Solid Edge part; units mm, degrees
sketch "Sketch1" plane through (0, 0, 0) normal (0, -1, 0) x (1, 0, 0)
  arc A0 (7.8125, -39.2296) -> (7.8125, 39.2296) centre (0, 0) cw
  arc A1 (7.8125, 39.2296) -> (242.1875, 39.2296) centre (125, 627.6743) ccw
  arc A2 (242.1875, 39.2296) -> (242.1875, -39.2296) centre (250, 0) cw
  arc A3 (242.1875, -39.2296) -> (7.8125, -39.2296) centre (125, -627.6743) ccw
  dimension "D1" = 39.2296
extrude "Protrusion1" add sketch "Sketch1" against normal blind 15
sketch "Sketch2" plane through (125, 0, 0) normal (0, -1, 0) x (1, 0, 0)
  circle A0 centre (125, 0) radius 22
extrude "Cutout1" cut sketch "Sketch2" against normal through all
hole "Agujero_1" at (250, 0, 32.5) direction (0, 1, 0) diameter 6.647 end up to next
pattern_circular "Pattern1" count 6 over 360 about axis through (250, 0, 0) along (0, 1, 0) of "Agujero_1"
sketch "Sketch3" plane through (125, 0, 0) normal (0, -1, 0) x (1, 0, 0)
  circle A0 centre (-125, 0) radius 3.2
extrude "Cutout2" cut sketch "Sketch3" against normal through all
sketch "Sketch4" plane through (125, 15, 0) normal (0, 1, 0) x (1, 0, 0)
  line L0 (-119, -6) -> (-131, -6)
  line L1 (-131, -6) -> (-131, 6)
  line L2 (-131, 6) -> (-119, 6)
  line L3 (-119, 6) -> (-119, -6)
  dimension "D1" = 131
  dimension "D2" = 119
extrude "VaciadoExtruido_3" cut sketch "Sketch4" against normal blind 12
sketch "Sketch5" plane through (125, 15, 0) normal (0, 1, 0) x (1, 0, 0)
  circle A0 centre (-125, 0) radius 20
extrude "VaciadoExtruido_4" cut sketch "Sketch5" against normal blind 3
hole "Agujero_7" at (-13, 0, 0) direction (0, 1, 0) diameter 4.5 end up to next counterbore diameter 8 counterbore depth 7
pattern_circular "Pattern2" count 6 over 360 about axis through (0, 0, 0) along (0, 1, 0) of "Agujero_7"
hole "Agujero_13" at (48.91, 0, 15) direction (0, 1, 0) diameter 6.647 end up to next
hole "Hole11" at (145.41, 0, 15) direction (0, 1, 0) diameter 6.647 end up to next
hole "Hole12" at (145.41, 0, -15) direction (0, 1, 0) diameter 6.647 end up to next
hole "Hole13" at (48.91, 0, -15) direction (0, 1, 0) diameter 6.647 end up to next
sketch "Sketch6" plane through (125, 0, 0) normal (0, -1, 0) x (1, 0, 0)
  line L0 (7.41, -22) -> (-63.09, -22)
  line L1 (-63.09, -22) -> (-63.09, 22)
  line L2 (-63.09, 22) -> (7.41, 22)
  line L3 (7.41, 22) -> (7.41, -22)
  dimension "D1" = 63.09
  dimension "D2" = 7.41
extrude "Cutout3" cut sketch "Sketch6" against normal through all
fillet "Redondeo_1" radius 5 4 edges at (61.91, 7.5, 22) (132.41, 7.5, 22) (61.91, 7.5, -22) (132.41, 7.5, -22)
For this review, take the finished solid that the model builds, in its own axes (mm). A direction names the side the tool comes from. Give positions to 0.01 mm unless a question says otherwise; leave off trailing zeros. Loops run counter-clockwise (first coordinate to the right, second up) from the corner with the lowest first, then second, coordinate; pieces in that order, holes last. Notation, with made-up numbers: M -4,83.25 L 17,83.25 A25 cw 17,105.25 Z; hole C -16.5,-9 d7. An arc over 180 degrees is marked long. Put each result on its own line as item: value. Start each with the question number.
(1) For pin 1 (2 mm diameter, centred on y = 11.5, z = 4, fed in from +X); pin 2 (6 mm diameter, centred on x = 47, y = 2, fed in from -Z); pin 3 (7.5 mm diameter, centred on x = 48.91, z = -15, fed in from -Y); pin 4 (2.5 mm diameter, centred on x = 8.5, z = -12.5, fed in from -Y), all flat-tipped, find the tip position at first contact; note any pin that passes through.
(2) Add section D-D, the plane x = 180.5. Write out the cut boundary in (y, z), then the cut area to 3 significant figures.
(3) Add section B-B, the plane x = 145.41. Write out the cut boundary in (y, z), then the cut area to 3 significant figures.
(4) Machinability: for faces 1 (the cylindrical face through (126.651, 7.395, -27.677)), 2 (the flat face through (4, 7, 11)), 3 (the flat face through (0, 8, 6)), 4 (the flat face through (132.41, 7, 0)), which of the approach directions +Z, -Z, +X, -X, +Y, -Y give a long, thin tool a straight path to every point of the face, cutting with its end or side? Answer none if there is none.
(5) Wall thickness on L1, parallel to Z at x = 250, y = 8.5; L2, parallel to Z at x = 48.91, y = 3.5; L3, parallel to Z at x = 8, y = 4.5: over which ranges is each line inside the solid? List them lowest first.
(6) Add section C-C, the plane z = 32.5. Write out the cut boundary in (x, y).
(7) Add section A-A, the plane x = 250. Write out the cut boundary in (y, z).
Result:
1. pin 1: stops at x = 289.89
1. pin 2: stops at z = -33.17
1. pin 3: stops at y = 0
1. pin 4: stops at y = 7
2. outline: M 0,-30.25 L 15,-30.25 L 15,30.25 L 0,30.25 Z
2. area: 907 mm^2
3. outline: M 0,-28.02 L 15,-28.02 L 15,-18.32 L 0,-18.32 Z; M 0,-11.68 L 15,-11.68 L 15,11.68 L 0,11.68 Z; M 0,18.32 L 15,18.32 L 15,28.02 L 0,28.02 Z
3. area: 641 mm^2
4. face 1: -Z, +Y, -Y
4. face 2: -Y
4. face 3: +Y
4. face 4: +Y, -Y
5. L1: z = -40 to -35.82, -29.18 to -22, 22 to 29.18, 35.82 to 40
5. L2: z = -32.52 to -18.32, -11.68 to 11.68, 18.32 to 32.52
5. L3: z = -39.19 to -14.97, -7.55 to 7.55, 14.97 to 39.19
6. outline: M -23.32,0 L 49.06,0 L 49.06,15 L -23.32,15 Z; M 200.94,0 L 246.68,0 L 246.68,15 L 200.94,15 Z; M 253.32,0 L 273.32,0 L 273.32,15 L 253.32,15 Z
7. outline: M 0,-40 L 15,-40 L 15,-35.82 L 0,-35.82 Z; M 0,-29.18 L 15,-29.18 L 15,-22 L 0,-22 Z; M 0,22 L 15,22 L 15,29.18 L 0,29.18 Z; M 0,35.82 L 15,35.82 L 15,40 L 0,40 Z
